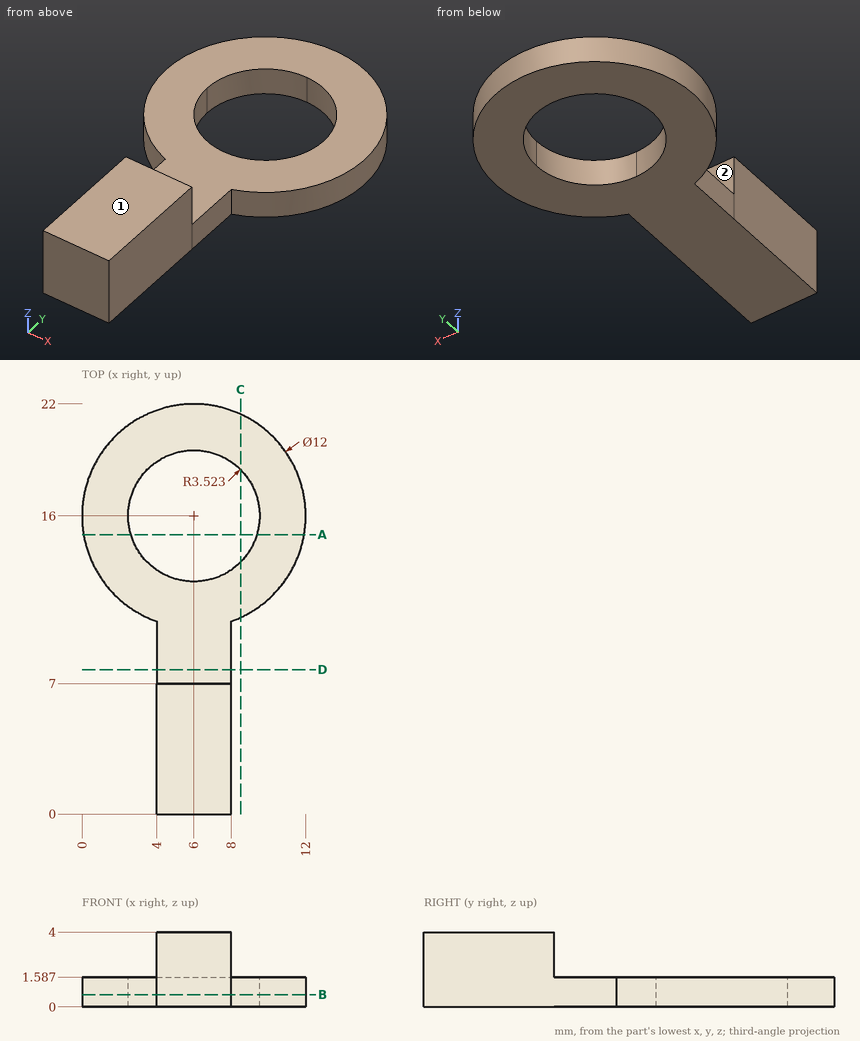
Answer from the drawing. Dimensions are ordinates in mm from the lowest x, y and z of the part. A direction names the side the tool comes from. Round coordinates to 2 decimals unless told otherwise and drop trailing zeros. Order: outer loops, then holes, each group sorted by start corner. A loop starts at its lowest first (then second) coordinate and runs counter-clockwise, first axis right, second up. Notation, with made-up numbers: (-16.75, 58.5) - (31.25, 58.5) arc R25 cw to (31.25, 74.5) - close; hole circle Ø7 at (57, 39). An arc over 180 degrees is marked (long way). Put each result on its own line as item: value. Start each with the question number.
(1) Given P1, Ø1, axis at y = 9.5, z = 2.5, coming from the -X side; P2, Ø2, axis at y = 4.5, z = 1, coming from the +X side; P3, Ø6, axis at x = 7.5, y = 14.5, coming from the +Z side; P4, Ø2, axis at x = 4, z = 1, coming from the +Y side, each flat-ended and moving along its own axis, determine where each tip first touches the part or whether it passes through.
(2) Find section B-B (z = 0.65). Give the vertices of the cut face in (x, y).
(3) Find section C-C (x = 8.5). Give the vertices of the cut face in (y, z) (1 decimal).
(4) Straight lines are drawn through the part: probe 1 along Z at (x, y) = (11, 18); probe 2 along Y at (x, z) = (6.5, 3.7); probe 3 along Y at (x, z) = (4.25, 1.4). For each, find the intervals that lie inside material, in ascending order. Write a range as from..to.
(5) Find section D-D (y = 7.75). Give the vertices of the cut face in (x, z).
(6) For the marked faces 1 and 2, determine the directions among +Z, -Z, +X, -X, +Y, -Y from which every point of the face is accessible in a straight line to the end or side of a thin tool.
(7) Find section A-A (y = 15). Give the vertices of the cut face in (x, z).
Reply:
1. P1: through
1. P2: x = 8
1. P3: z = 1.59
1. P4: y = 21.92
2. outline: (4, 0) - (8, 0) - (8, 10.34) arc R6 ccw (long way) to (4, 10.34) - close; hole circle Ø7.05 at (6, 16)
3. outline: (10.5, 0) - (13.5, 0) - (13.5, 1.6) - (10.5, 1.6) - close; (18.5, 0) - (21.5, 0) - (21.5, 1.6) - (18.5, 1.6) - close
4. probe 1: 0..1.59
4. probe 2: 0..7
4. probe 3: 0..12.94, 19.06..21.74
5. outline: (4, 0) - (8, 0) - (8, 1.59) - (4, 1.59) - close
6. face 1: +Z, +X, -X, +Y, -Y
6. face 2: +Z, +X, -X, +Y
7. outline: (0.08, 0) - (2.62, 0) - (2.62, 1.59) - (0.08, 1.59) - close; (9.38, 0) - (11.92, 0) - (11.92, 1.59) - (9.38, 1.59) - close
